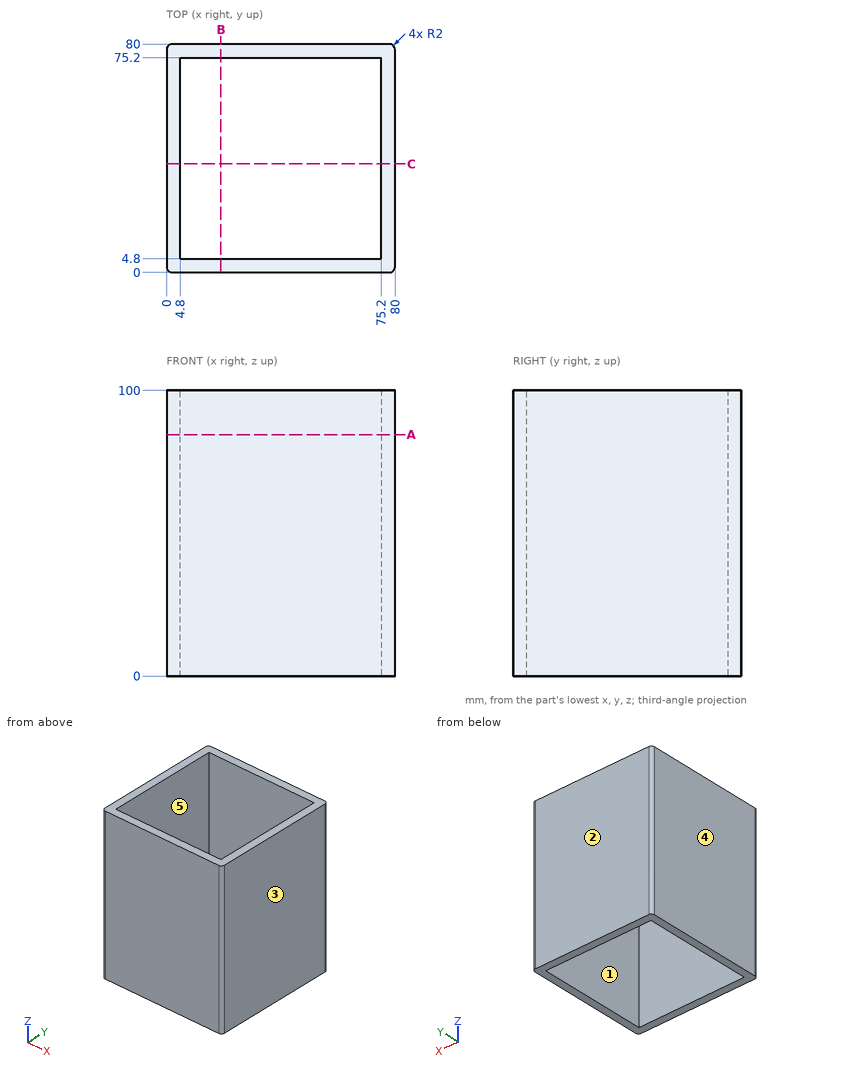
Check sheet for the drawn part. Datum: minimum x, y, z corner. Units: mm. A direction names the side the tool comes from. Give positions to 0.01 mm unless a question says otherwise; leave off trailing zeros. Write each loop counter-clockwise with the first axis right and the second up, starting at its lowest first coordinate (ties: lowest second). Pieces come first, ordered by that corner, then holes.
(1) Access from +Z, -Z, +X, -X, +Y, -Y to the whole of each face (thin tool, end or side, straight path). Record for the marked faces 4 and 5.
(2) Mould release check, pull along Y, two halves, no side actions. Record for the marked faces 1, 2 and 3: +Y half, -Y half, draft (parallel to the pull), parting line (faces both ways), or undercut.
(3) Cross-section at B-B (x = 19). Enter the section's corners in (y, z).
(4) Material ranges on line 1 (Y direction, x = 24, z = 58), recorded low to high.
(5) Cross-section at A-A (z = 84.5). Enter the section's corners in (x, y).
Worked out:
1. face 4: +Z, -Z, -X, +Y, -Y
1. face 5: +Z, -Z
2. face 1: undercut
2. face 2: +Y half
2. face 3: draft
3. outline: (0, 0) - (4.8, 0) - (4.8, 100) - (0, 100) - close; (75.2, 0) - (80, 0) - (80, 100) - (75.2, 100) - close
4. line 1: y = 0 to 4.8, 75.2 to 80
5. outline: (0, 2) arc R2 ccw to (2, 0) - (78, 0) arc R2 ccw to (80, 2) - (80, 78) arc R2 ccw to (78, 80) - (2, 80) arc R2 ccw to (0, 78) - close; hole (4.8, 4.8) - (75.2, 4.8) - (75.2, 75.2) - (4.8, 75.2) - close
